For this review, take the finished solid that the model builds, in its own axes (mm). Give positions to 0.01 mm unless a question says otherwise; leave off trailing zeros. Order: outer loops, then holes, each group sorted by start corner. A loop starts at its lowest first (then second) coordinate and runs counter-clockwise, first axis right, second up. Notation, with made-up numbers: (35.5, 16.5) -> (72.5, 16.5) arc R23 ccw to (72.5, 53.5) -> close; hole circle Ø5 at (16, -31.5). An arc over 180 degrees is marked (long way). Use CSV: the item, a comma, the result in double quotes. Start each with the question number.
```python
from build123d import *

# Parameters (mm, degrees)
SKETCH1_R           = 3.175
BOSS_EXTRUDE1_DEPTH = 330.2
SKETCH2_R           = 3.4925
SKETCH2_R_2         = 2.38125
CUT_EXTRUDE1_DEPTH  = 3.96875
LPATTERN1_COUNT     = 2
LPATTERN1_PITCH     = 107.95


with BuildPart() as part:
    # Sketch1 → Boss-Extrude1 (new body)
    with BuildSketch(Plane(origin=(0, 0, 0), x_dir=(1, 0, 0), z_dir=(0, 1, 0))):
        with Locations(Location((0, 0, 0), (0, 0, 270))):  # turned: the seam where the file's is
            Circle(SKETCH1_R)
    extrude(amount=BOSS_EXTRUDE1_DEPTH)

    # Sketch2 → Cut-Extrude1 (cut)
    with BuildSketch(Plane(origin=(0, 108.83011, 0), x_dir=(-1, 0, 0), z_dir=(0, 1, 0))):
        Circle(SKETCH2_R)
        with Locations(Location((0, 0, 0), (0, 0, 90))):  # turned: the seam where the file's is
            Circle(SKETCH2_R_2, mode=Mode.SUBTRACT)
    cut_extrude1 = extrude(amount=CUT_EXTRUDE1_DEPTH, mode=Mode.SUBTRACT)

    # LPattern1: Cut-Extrude1 ×2
    with Locations(*[(0, i * LPATTERN1_PITCH, 0) for i in range(1, LPATTERN1_COUNT)]):
        add(cut_extrude1, mode=Mode.SUBTRACT)


solid = part.part
```
1. Draft analysis for pull direction Y (two halves, no side actions). For faces 1 (the face through (-1.93, 274.71, -2.52)), 2 (the face through (0, 330.2, 0)), 3 (the face through (0, 0, 0)), state which applies: +Y half, -Y half, draft (parallel to the pull), parting line (faces both ways), or undercut.
2. To check wall thickness, follow L1, parallel to Y at x = 0.5, z = 2.5; L2, parallel to X at y = 224.5, z = -0.5; L3, parallel to Z at x = -0.25, y = 155.5. State the ranges of each line that lie inside material, in increasing order. Write a range as [from, to].
3. Clearance check with a flat-ended pin moving along its axis: P1, Ø3, axis at x = -2.5, y = 136.5, coming from the -Z side. State where the tip first meets the part, or that it passes through.
4. Consider section C-C (y = 263.5). State the section outline as (x, z) points (3 decimals).
5. Consider section B-B (x = 1). State the section outline as (y, z) points, plus the area to 3 significant figures.
6. Consider section A-A (z = 1). State the section outline as (x, y) points, plus the area to 3 significant figures.
Answer list:
1,face 1,"draft"
1,face 2,"+Y half"
1,face 3,"-Y half"
2,L1,"[0, 108.83], [112.8, 216.78], [220.75, 330.2]"
2,L2,"[-3.14, 3.14]"
2,L3,"[-3.17, 3.17]"
3,P1,"z = -3.01"
4,outline,"circle Ø6.35 at (0, 0)"
5,outline,"(0, -3.01) -> (108.83, -3.01) -> (108.83, -2.16) -> (112.8, -2.16) -> (112.8, -3.01) -> (216.78, -3.01) -> (216.78, -2.16) -> (220.75, -2.16) -> (220.75, -3.01) -> (330.2, -3.01) -> (330.2, 3.01) -> (220.75, 3.01) -> (220.75, 2.16) -> (216.78, 2.16) -> (216.78, 3.01) -> (112.8, 3.01) -> (112.8, 2.16) -> (108.83, 2.16) -> (108.83, 3.01) -> (0, 3.01) -> close"
5,area,"1,980 mm2"
6,outline,"(-3.01, 0) -> (3.01, 0) -> (3.01, 108.83) -> (2.16, 108.83) -> (2.16, 112.8) -> (3.01, 112.8) -> (3.01, 216.78) -> (2.16, 216.78) -> (2.16, 220.75) -> (3.01, 220.75) -> (3.01, 330.2) -> (-3.01, 330.2) -> (-3.01, 220.75) -> (-2.16, 220.75) -> (-2.16, 216.78) -> (-3.01, 216.78) -> (-3.01, 112.8) -> (-2.16, 112.8) -> (-2.16, 108.83) -> (-3.01, 108.83) -> close"
6,area,"1,980 mm2"
